Could you check a few things on this model? Use its own coordinates, in mm. Face numbers are marked on the shaded views. A direction names the side the tool comes from. Round coordinates to 2 decimals unless told otherwise and drop trailing zeros. Order: outer loops, then holes, each group sorted by start corner. A loop starts at its lowest first (then second) coordinate and runs counter-clockwise, first axis right, second up. Notation, with made-up numbers: M 87,11.25 L 129,11.25 A9 cw 129,17.25 Z; hole C 35.5,43 d5. An arc over 180 degrees is marked long. Write each question's results on one line, items separated by ' | '. Start each with the question number.
1. For the marked faces 1 and 2, which set-ups out of +Z, -Z, +X, -X, +Y, -Y let a thin tool reach every point of the face, with its end or its side?
2. Please list where these lines run through material, in increasing order: L1, parallel to X at y = -0.05, z = 28.2; L2, parallel to Z at x = -36, y = -11.5; L3, parallel to Z at x = -11, y = -26.
3. I'm going to push flat-ended pins straight in: pin 1 (1.5 mm diameter, centred on x = 1, y = 36.5, fed in from +Z); pin 2 (8 mm diameter, centred on y = -13, z = 55, fed in from -X); pin 3 (1.6 mm diameter, centred on x = 37, y = 0, fed in from +Z); pin 4 (2 mm diameter, centred on x = -36.22, z = 28.2, fed in from +Y). Where does each tip first touch, or does it pass through?
4. Suppose I cut it at C-C on z = 66.5. Write out the boundary of the cut face in (x, y).
from build123d import *

# Parameters (mm, degrees)
SKETCH3_W           = 2
SKETCH3_H           = 13.6
BOSS_EXTRUDE1_DEPTH = 39.25
SKETCH4_R           = 1.25
CUT_EXTRUDE1_DEPTH  = 113.281176072
SKETCH5_R           = 1.5
BOSS_EXTRUDE5_DEPTH = 50


with BuildPart() as part:
    # Sketch1 → Revolve1 (revolve)
    with BuildSketch(Plane.YZ, mode=Mode.PRIVATE) as revolve1_sk:
        Polygon((0, 0), (38.5, 0), (38.5, 2), (36.2, 2), (33.6, 8.225), (33.6, 21.4), (33.2, 21.4), (33.2, 45), (5, 45), (5, 46), (12, 46), (14, 48.25), (14, 86.25), (12, 88.5), (2, 88.5), (2, 97.5), (0, 97.5), align=None)
    revolve(revolve1_sk.sketch.rotate(Axis((0, 0, 0), (0, 0, -1)), 90), axis=Axis((0, 0, 0), (0, 0, -1)))

    # Sketch3 → Boss-Extrude1 (add, symmetric)
    with BuildSketch(Plane.YZ):
        with Locations((0, 28.2)):
            Rectangle(SKETCH3_W, SKETCH3_H)
    extrude(amount=BOSS_EXTRUDE1_DEPTH, both=True)

    # Sketch4 → Cut-Extrude1 (cut, through all)
    with BuildSketch(Plane(origin=(0, 1, 0), x_dir=(-1, 0, 0), z_dir=(0, 1, 0))):
        with Locations(Location((-36.217468171, 28.2, 0), (0, 0, 90))):
            Circle(SKETCH4_R)
    cut_extrude1 = extrude(amount=-CUT_EXTRUDE1_DEPTH, mode=Mode.SUBTRACT)

    # Mirror1: Cut-Extrude1 across plane
    add(cut_extrude1.mirror(Plane(origin=(0, 0, 0), x_dir=(0, 0, 1), z_dir=(1, 0, 0))), mode=Mode.SUBTRACT)

    # Sketch5 → Boss-Extrude5 (add)
    with BuildSketch(Plane(origin=(0, 0, 0), x_dir=(-1, 0, 0), z_dir=(0, 1, 0))):
        with Locations(Location((0, 48, 0), (0, 0, 9.594065947))):
            Circle(SKETCH5_R)
        with Locations(Location((4, 48, 0), (0, 0, 170.405931773))):
            Circle(SKETCH5_R)
        with Locations(Location((-4, 48, 0), (0, 0, 170.405931773))):
            Circle(SKETCH5_R)
    extrude(amount=BOSS_EXTRUDE5_DEPTH)


solid = part.part
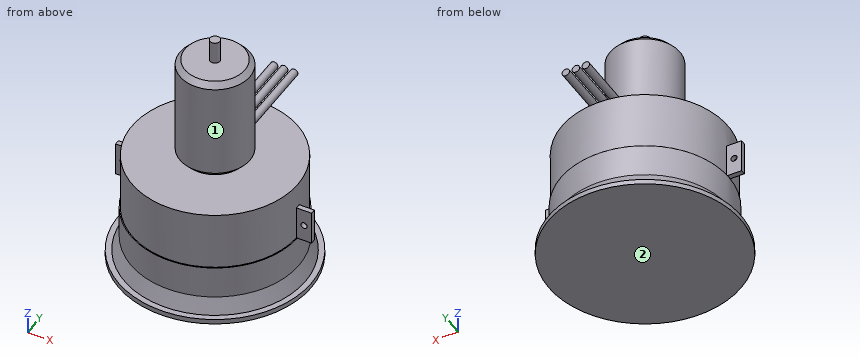
Filled sheet:
1) face 1: +Z | face 2: -Z, +X, -X, +Y, -Y
2) L1: x = -39.25 to -37.47, -34.97 to 34.97, 37.47 to 39.25 | L2: z = 0 to 2 | L3: z = 0 to 45
3) pin 1: stops at z = 49.48 | pin 2: stops at x = -10.72 | pin 3: stops at z = 35 | pin 4: passes through
4) outline: C 0,0 d28
